Verification items for the finished model (mm, model axes). A direction names the side the tool comes from. Give positions to 0.01 mm unless a question says otherwise; leave off trailing zeros. Write each loop counter-clockwise with the first axis right and the second up, starting at its lowest first coordinate (ties: lowest second). Pieces come first, ordered by that corner, then holes. Notation, with made-up numbers: (20.5, -3.5) - (61.5, -3.5) arc R17 ccw to (61.5, 5.5) - close; hole circle Ø5 at (78, -27). An arc over 180 degrees is marked (long way). Put each result on its own line as item: value.
from build123d import *

# Parameters (mm, degrees)
CROQUIS2_R                 = 30
SALIENTE_EXTRUIR1_DEPTH    = 60
CROQUIS3_W                 = 40
CROQUIS3_H                 = 30
SALIENTE_EXTRUIR2_DEPTH    = 30
REDONDEO1_R                = 10
CROQUIS4_R                 = 5
CORTAR_EXTRUIR1_DEPTH      = 81.777472107
CORTAR_EXTRUIR2_DEPTH      = 74.484692283
CORTAR_EXTRUIR2_DEPTH_BACK = 74.484692283
CROQUIS7_R                 = 25
CORTAR_EXTRUIR3_DEPTH      = 70.462219947
CROQUIS8_R                 = 5
CROQUIS8_R_2               = 10
SALIENTE_EXTRUIR3_DEPTH    = 200
CROQUIS10_R                = 23.462912018
SALIENTE_EXTRUIR4_DEPTH    = 5
CROQUIS11_R                = 2.5
SALIENTE_EXTRUIR5_DEPTH    = 5


with BuildPart() as part:
    # Croquis2 → Saliente-Extruir1 (new body)
    with BuildSketch(Plane(origin=(0, 0, 0), x_dir=(1, 0, 0), z_dir=(0, 1, 0))):
        with Locations(Location((0, 0, 0), (0, 0, 270))):
            Circle(CROQUIS2_R)
    extrude(amount=SALIENTE_EXTRUIR1_DEPTH)

    # Croquis3 → Saliente-Extruir2 (add)
    with BuildSketch(Plane.XZ):
        Rectangle(CROQUIS3_W, CROQUIS3_H)
    extrude(amount=SALIENTE_EXTRUIR2_DEPTH)

    # Redondeo1
    redondeo1_edges = [part.edges().sort_by_distance(p)[0] for p in [
        (-20, -30, 0),
        (20, -30, 0),
    ]]
    fillet(redondeo1_edges, radius=REDONDEO1_R)

    # Croquis4 → Cortar-Extruir1 (cut, through all)
    with BuildSketch(Plane.XY.offset(15)):
        with Locations((0, -20)):
            Circle(CROQUIS4_R)
    extrude(amount=-CORTAR_EXTRUIR1_DEPTH, mode=Mode.SUBTRACT)

    # Croquis5 → Cortar-Extruir2 (cut, two sides: drawn at the far end of the back side and taken through both)
    with BuildSketch(Plane.XY.offset(-CORTAR_EXTRUIR2_DEPTH_BACK)):
        Polygon((30, 60), (-30, 60), (30, 25.358983849), align=None)
    extrude(amount=CORTAR_EXTRUIR2_DEPTH + CORTAR_EXTRUIR2_DEPTH_BACK, mode=Mode.SUBTRACT)

    # Croquis7 → Cortar-Extruir3 (cut, through all)
    with BuildSketch(Plane(origin=(0, 5, 0), x_dir=(-1, 0, 0), z_dir=(0, -1, 0))):
        with Locations(Location((0, 0, 0), (0, 0, 90))):
            Circle(CROQUIS7_R)
    extrude(amount=-CORTAR_EXTRUIR3_DEPTH, mode=Mode.SUBTRACT)

    # Croquis8 → Saliente-Extruir3 (add)
    with BuildSketch(Plane(origin=(0, 5, 0), x_dir=(1, 0, 0), z_dir=(0, 1, 0))):
        with Locations(Location((0, 16.650635095, 0), (0, 0, 90))):
            Circle(CROQUIS8_R)
        with Locations(Location((12.5, -5, 0), (0, 0, 90))):
            Circle(CROQUIS8_R_2)
        with Locations(Location((-12.5, -5, 0), (0, 0, 90))):
            Circle(CROQUIS8_R)
    extrude(amount=SALIENTE_EXTRUIR3_DEPTH)

    # Croquis10 → Saliente-Extruir4 (add)
    with BuildSketch(Plane(origin=(0, 205, 0), x_dir=(1, 0, 0), z_dir=(0, 1, 0))):
        with Locations(Location((0, 0, 0), (0, 0, 338.198590514))):
            Circle(CROQUIS10_R)
    extrude(amount=SALIENTE_EXTRUIR4_DEPTH)

    # Croquis11 → Saliente-Extruir5 (add, symmetric)
    with BuildSketch(Plane(origin=(0, 0, 0), x_dir=(-1, 0, 0), z_dir=(0, 0, -1))):
        with BuildLine():
            Line((-27.185083119, -44.006420995), (-20, -20))
            Line((-20, -20), (0.452470226, -27.989728354))
            Line((0.452470226, -27.989728354), (20, -18.654592883))
            Line((20, -18.654592883), (26.768433701, -32.834107425))
            ThreePointArc((26.768433701, -32.834107425), (26.788350186, -39.25372151), (21.834748215, -43.337061956))
            Line((21.834748215, -43.337061956), (-18.165251785, -53.42902271))
            ThreePointArc((-18.165251785, -53.42902271), (-25.417829516, -51.343148457), (-27.185083119, -44.006420995))
        make_face()
        with Locations((-20, -46.156904794)):
            Circle(CROQUIS11_R, mode=Mode.SUBTRACT)
        with Locations((20, -36.06494404)):
            Circle(CROQUIS11_R, mode=Mode.SUBTRACT)
    extrude(amount=SALIENTE_EXTRUIR5_DEPTH, both=True)


solid = part.part
Q1. Section check B-B, the plane x = 0. Record the cut outline in (y, z).
Answers follow:
outline: (-48.85, -5) - (-30, -5) - (-30, -15) - (-25, -15) - (-25, 15) - (-30, 15) - (-30, 5) - (-48.85, 5) - close; (-15, -15) - (0, -15) - (0, -30) - (42.68, -30) - (42.68, -25) - (5, -25) - (5, -21.65) - (205, -21.65) - (205, -23.46) - (210, -23.46) - (210, 23.46) - (205, 23.46) - (205, -11.65) - (5, -11.65) - (5, 25) - (42.68, 25) - (42.68, 30) - (0, 30) - (0, 15) - (-15, 15) - close
Q2. Go/stop test with flat-tipped pins: pin 1 Ø2 at (x, z) = (0.5, -15) entering from -Y; pin 2 Ø8 at (y, z) = (46, 10.5) entering from -X; pin 3 Ø18 at (x, z) = (-3.5, -11.5) entering from -Y; pin 4 Ø8 at (x, y) = (0, -20) entering from -Z. Record where each tip stops, or that it passes through.
Answers follow:
pin 1: stops at y = -30
pin 2: stops at x = -29.29
pin 3: stops at y = -49.53
pin 4: passes through
Q3. Section check D-D, the plane y = -4.5. Record the cut outline in (x, z), plus the area to 3 significant figures.
Answers follow:
outline: (-20, -15) - (20, -15) - (20, 15) - (-20, 15) - close
area: 1,200 mm2
Q4. Section check C-C, the plane x = -12.5. Record the cut outline in (y, z), plus the area to 3 significant figures.
Answers follow:
outline: (-45.69, -5) - (-29.68, -5) - (-29.68, -15) - (0, -15) - (0, -27.27) - (49.9, -27.27) - (49.9, -21.65) - (5, -21.65) - (5, 0) - (205, 0) - (205, -19.86) - (210, -19.86) - (210, 19.86) - (205, 19.86) - (205, 10) - (5, 10) - (5, 21.65) - (49.9, 21.65) - (49.9, 27.27) - (0, 27.27) - (0, 15) - (-29.68, 15) - (-29.68, 5) - (-45.69, 5) - close
area: 4,030 mm2
Q5. Scan lines: line 1 along Y through (x, z) = (-8, -18.5); line 2 along Z through (x, y) = (-3.5, 12.5); line 3 along Y through (x, z) = (0, -1.25). Record each from-to range of solid material in increasing order.
Answers follow:
line 1: y = 0 to 5, 205 to 210
line 2: z = -29.8 to -24.75, -20.22 to -13.08, 24.75 to 29.8
line 3: y = -48.85 to -25, -15 to 5, 205 to 210
Q6. Section check A-A, the plane y = 77.5. Record the cut outline in (x, z), plus the area to 3 significant figures.
Answers follow:
outline: circle Ø10 at (-12.5, 5); circle Ø10 at (0, -16.65); circle Ø20 at (12.5, 5)
area: 471 mm2
Q7. Set-up check for faces 1 (the face through (23.643, -32.171, -0.07)), 2 (the face through (-17.15, -26.99, 10.07)), 3 (the face through (17.15, -26.99, -9.93)): record each of +Z, -Z, +X, -X, +Y, -Y from which the full face is reachable in a straight line by a thin tool's end or side.
Answers follow:
face 1: +Z, -Z, +X
face 2: +Z, -X, -Y
face 3: -Z, +X, -Y
Q8. Release check for a two-part mould opening along Y. For faces 4 (the face through (21.372, 103.6, 0.386)), 5 (the face through (0, -30, 10)), 6 (the face through (20, -10, 0)), 7 (the face through (-0.3, -14.8, 15)) record: released by +Y, released by -Y, zero draft, split by the parting line, or undercut.
Answers follow:
face 4: undercut
face 5: released by -Y
face 6: undercut
face 7: zero draft
